For this review, take the finished solid that the model builds, in its own axes (mm). Give positions to 0.01 mm unless a question says otherwise; leave off trailing zeros.
1) For P1, Ø0.5, axis at y = 26, z = 37, coming from the -X side; P2, Ø4.5, axis at x = 104.775, z = 28.575, coming from the -Y side; P3, Ø0.5, axis at y = 26.5, z = 35.5, coming from the +X side, all flat-tipped, find the tip position at first contact; note any pin that passes through.
2) Draft analysis for pull direction X (two halves, no side actions). For faces 1 (the face through (151.107, 26.183, 28.328)), 2 (the face through (138, 25.4, 1)), state which applies: pulls with the +X half, pulls with the -X half, needs draft (parallel to the pull), parting line crosses it, or undercut.
3) Wall thickness on line 1 along Z through (x, y) = (149, 25.95); line 2 along X through (y, z) = (26.5, -28.5); line 3 along Z through (x, y) = (106.5, 26.3): over which ranges is each line inside the solid? List them lowest first.
4) We need section A-A on y = 26. Give the number of separate pieces and of enclosed holes in the cut face, and give its area (3 significant figures).
from build123d import *

# Parameters (mm, degrees)
BOSS_EXTRUDE1_DEPTH   = 25.4
SKETCH4_W             = 63.5
SKETCH4_H             = 76.2
CUT_EXTRUDE4_DEPTH    = 0.01
F_6_CLEARANCE_HOLE1_D = 3.7973
CUT_EXTRUDE5_DEPTH    = 3.5052
SKETCH8_R             = 1.89865
BOSS_EXTRUDE2_DEPTH   = 1.5875
SKETCH9_W             = 83.512513563
SKETCH9_H             = 26.66457596
CUT_EXTRUDE7_DEPTH    = 309.355274367
SKETCH10_W            = 76.2
SKETCH10_H            = 78.034990754
SKETCH10_W_2          = 120.649995745
SKETCH10_H_2          = 89.760717872
CUT_EXTRUDE8_DEPTH    = 305.02593568


with BuildPart() as part:
    # Sketch1 → Boss-Extrude1 (new body)
    with BuildSketch(Plane(origin=(0, 0, 0), x_dir=(1, 0, 0), z_dir=(0, 1, 0))):
        with BuildLine():
            Line((76.2, 38.1), (177.8, 38.1))
            add(Edge.make_bspline(
                [(177.8, -38.1), (304.8, -38.1), (304.8, 0), (304.8, 38.1), (177.8, 38.1)],
                knots=[4.71238898, 4.71238898, 4.71238898, 6.283185307, 6.283185307, 7.853981634, 7.853981634, 7.853981634], degree=2, weights=[1, 0.707106781, 1, 0.707106781, 1]))
            Line((177.8, -38.1), (76.2, -38.1))
            add(Edge.make_bspline(
                [(76.2, 38.1), (0, 38.1), (0, 0), (0, -38.1), (76.2, -38.1)],
                knots=[4.71238898, 4.71238898, 4.71238898, 6.283185307, 6.283185307, 7.853981634, 7.853981634, 7.853981634], degree=2, weights=[1, 0.707106781, 1, 0.707106781, 1]))
        make_face()
    extrude(amount=BOSS_EXTRUDE1_DEPTH)

    # Sketch4 → Cut-Extrude4 (cut)
    with BuildSketch(Plane.XZ):
        with Locations((107.95, 0)):
            Rectangle(SKETCH4_W, SKETCH4_H)
    extrude(amount=-CUT_EXTRUDE4_DEPTH, mode=Mode.SUBTRACT)

    # #6 Clearance Hole1 (through all)
    with Locations(Plane(origin=(0, 25.4, 0), x_dir=(1, 0, 0), z_dir=(0, 1, 0))):
        with Locations((104.775, 28.575), (149.225, 28.575), (149.225, -28.575), (104.775, -28.575)):
            Hole(F_6_CLEARANCE_HOLE1_D / 2)

    # Sketch7 → Cut-Extrude5 (cut)
    with BuildSketch(Plane(origin=(0, 25.4, 0), x_dir=(1, 0, 0), z_dir=(0, 1, 0))):
        Polygon((144.092356107, 28.575), (146.658678053, 24.13), (151.791321947, 24.13), (154.357643893, 28.575), (151.791321947, 33.02), (146.658678053, 33.02), align=None)
        Polygon((144.092356107, -28.575), (146.658678053, -33.02), (151.791321947, -33.02), (154.357643893, -28.575), (151.791321947, -24.13), (146.658678053, -24.13), align=None)
        Polygon((99.642356107, -28.575), (102.208678053, -33.02), (107.341321947, -33.02), (109.907643893, -28.575), (107.341321947, -24.13), (102.208678053, -24.13), align=None)
        Polygon((99.642356107, 28.575), (102.208678053, 24.13), (107.341321947, 24.13), (109.907643893, 28.575), (107.341321947, 33.02), (102.208678053, 33.02), align=None)
    extrude(amount=-CUT_EXTRUDE5_DEPTH, mode=Mode.SUBTRACT)

    # Sketch8 → Boss-Extrude2 (add)
    with BuildSketch(Plane(origin=(0, 25.4, 0), x_dir=(1, 0, 0), z_dir=(0, 1, 0))):
        with BuildLine():
            Line((76.2, 34.925), (76.2, 38.1))
            Line((76.2, 38.1), (177.8, 38.1))
            Line((177.8, 38.1), (177.8, 34.925))
            add(Edge.make_bspline(
                [(177.8, -34.925), (183.4037084, -34.925), (188.998492342, -34.813401269), (200.169898566, -34.363095557), (205.746528757, -34.024487469), (216.880255629, -33.103008305), (222.437375795, -32.520430902), (230.75625716, -31.436497802), (233.526404303, -31.040006826), (239.060480939, -30.169274267), (241.826062226, -29.694714405), (250.088902803, -28.143630441), (255.558584053, -26.942274462), (262.328557631, -25.151722447), (263.679135198, -24.778907782), (266.372677584, -24.000520191), (267.71682163, -23.594573907), (271.725857042, -22.324580042), (274.36743953, -21.409387606), (279.569151408, -19.39956311), (282.129804397, -18.306084526), (285.88296458, -16.472402408), (287.119225286, -15.828587024), (289.55372457, -14.457194234), (290.752112946, -13.729946828), (293.096789788, -12.16067691), (294.246150852, -11.316137328), (295.874693947, -9.951173652), (296.402758109, -9.47890107), (297.421867434, -8.491073847), (297.913370929, -7.974720766), (298.834097865, -6.902845016), (299.265206405, -6.34585568), (300.051083084, -5.176943461), (300.406626859, -4.564345705), (301.008906586, -3.265877479), (301.246986609, -2.597792892), (301.485043085, -1.560074348), (301.544634961, -1.206113764), (301.617830117, -0.494585391), (301.644885041, 0.214202137), (301.581423052, 0.917612733), (301.474094585, 1.618417551), (301.397802992, 1.969801613), (301.111287523, 3.001503382), (300.846416268, 3.65704054), (300.206739898, 4.920093421), (299.828668717, 5.531043925), (299.007148253, 6.686383823), (298.562585264, 7.234082094), (297.622788002, 8.284550248), (297.127404223, 8.787187569), (296.096077792, 9.756500131), (295.558527194, 10.224239157), (293.916424424, 11.566158841), (292.777517596, 12.385848353), (290.439906756, 13.923799855), (289.240807105, 14.641390764), (286.797257835, 15.999650314), (285.552669877, 16.640084306), (283.027180157, 17.859357093), (281.744712958, 18.438732265), (279.156163214, 19.543403236), (277.854905585, 20.066703794), (273.933809615, 21.564574536), (271.296832059, 22.467878334), (265.988924804, 24.133309881), (263.317871138, 24.894922167), (255.263773486, 27.00954075), (249.84032756, 28.194552175), (238.914613399, 30.236824809), (233.411910816, 31.092279963), (225.108785934, 32.171421056), (222.333695526, 32.496639974), (216.783621708, 33.081533661), (214.006661761, 33.341462159), (205.670357358, 34.029518973), (200.105614733, 34.366364864), (188.962770448, 34.814156957), (183.384662687, 34.925), (177.8, 34.925)],
                knots=[0, 0, 0, 0, 0.0625, 0.0625, 0.125, 0.125, 0.1875, 0.1875, 0.21875, 0.21875, 0.25, 0.25, 0.3125, 0.3125, 0.328125, 0.328125, 0.34375, 0.34375, 0.375, 0.375, 0.40625, 0.40625, 0.421875, 0.421875, 0.4375, 0.4375, 0.453125, 0.453125, 0.4609375, 0.4609375, 0.46875, 0.46875, 0.4765625, 0.4765625, 0.484375, 0.484375, 0.4921875, 0.4921875, 0.49609375, 0.49609375, 0.5, 0.50390625, 0.50390625, 0.5078125, 0.5078125, 0.515625, 0.515625, 0.5234375, 0.5234375, 0.53125, 0.53125, 0.5390625, 0.5390625, 0.546875, 0.546875, 0.5625, 0.5625, 0.578125, 0.578125, 0.59375, 0.59375, 0.609375, 0.609375, 0.625, 0.625, 0.65625, 0.65625, 0.6875, 0.6875, 0.75, 0.75, 0.8125, 0.8125, 0.84375, 0.84375, 0.875, 0.875, 0.9375, 0.9375, 1, 1, 1, 1], degree=3))
            Line((177.8, -34.925), (177.8, -38.1))
            Line((177.8, -38.1), (76.2, -38.1))
            Line((76.2, -38.1), (76.2, -34.925))
            add(Edge.make_bspline(
                [(76.2, 34.925), (72.560356463, 34.925), (68.943360269, 34.792561899), (61.754441862, 34.264100128), (58.182504946, 33.868162444), (51.086537454, 32.796138329), (47.562444107, 32.120418968), (40.569083399, 30.448366491), (37.099631765, 29.453110976), (32.806027277, 27.95635597), (31.949494882, 27.644206952), (30.241174952, 26.992161717), (29.390926264, 26.65279755), (26.866144113, 25.597394738), (25.212373464, 24.842354074), (21.972821409, 23.213388071), (20.386939209, 22.339638978), (17.297386897, 20.44838632), (15.793478172, 19.43129999), (13.617299122, 17.766336528), (12.904682274, 17.187440617), (11.513561893, 15.976499308), (10.840880513, 15.349552385), (9.54783147, 14.046551814), (8.927423545, 13.37053596), (8.042889277, 12.313259261), (7.755748062, 11.953602405), (7.198395375, 11.218396794), (6.928446634, 10.843070732), (5.637961842, 8.942133597), (4.781011076, 7.331767424), (4.011479694, 5.164717753), (3.872393075, 4.721427518), (3.630991775, 3.828466268), (3.528746677, 3.379752125), (3.278693467, 2.026749947), (3.187494563, 1.115610982), (3.170545544, -0.265601808), (3.185103724, -0.730659272), (3.254432294, -1.653608423), (3.308896513, -2.110722742), (3.528648511, -3.46965449), (3.750177803, -4.359086655), (4.185155464, -5.670622337), (4.348017487, -6.105682935), (4.702753212, -6.959314098), (4.89428858, -7.377540069), (5.507317523, -8.608922615), (5.967053776, -9.398893053), (6.972472791, -10.926725455), (7.518232478, -11.66454078), (8.684660756, -13.094754944), (9.299817788, -13.780178654), (11.212125162, -15.748333857), (12.581059513, -16.950990578), (14.739480167, -18.63278064), (15.476712229, -19.172714409), (16.982909755, -20.215658543), (17.753757316, -20.719762644), (20.090686263, -22.170309278), (21.683208327, -23.057695262), (26.543466505, -25.529337744), (29.892801319, -26.925597609), (35.037930237, -28.740921547), (36.773547574, -29.298627898), (39.40495658, -30.070716914), (40.286457068, -30.317183729), (42.05035166, -30.787397156), (42.933764127, -31.011448076), (47.357777286, -32.079253653), (50.919045806, -32.767054426), (58.079539287, -33.856246888), (61.678822068, -34.257202279), (68.912834907, -34.79163745), (72.5475805, -34.925), (76.2, -34.925)],
                knots=[0, 0, 0, 0, 0.0625, 0.0625, 0.125, 0.125, 0.1875, 0.1875, 0.25, 0.25, 0.265625, 0.265625, 0.28125, 0.28125, 0.3125, 0.3125, 0.34375, 0.34375, 0.375, 0.375, 0.390625, 0.390625, 0.40625, 0.40625, 0.421875, 0.421875, 0.4296875, 0.4296875, 0.4375, 0.4375, 0.46875, 0.46875, 0.4765625, 0.4765625, 0.484375, 0.484375, 0.5, 0.5, 0.5078125, 0.5078125, 0.515625, 0.515625, 0.53125, 0.53125, 0.5390625, 0.5390625, 0.546875, 0.546875, 0.5625, 0.5625, 0.578125, 0.578125, 0.59375, 0.59375, 0.625, 0.625, 0.640625, 0.640625, 0.65625, 0.65625, 0.6875, 0.6875, 0.75, 0.75, 0.78125, 0.78125, 0.796875, 0.796875, 0.8125, 0.8125, 0.875, 0.875, 0.9375, 0.9375, 1, 1, 1, 1], degree=3))
        make_face()
        with Locations(Location((149.225, 28.575, 0), (0, 0, 270))):
            Circle(SKETCH8_R, mode=Mode.SUBTRACT)
        with Locations(Location((149.225, -28.575, 0), (0, 0, 270))):
            Circle(SKETCH8_R, mode=Mode.SUBTRACT)
        with Locations(Location((104.775, -28.575, 0), (0, 0, 270))):
            Circle(SKETCH8_R, mode=Mode.SUBTRACT)
        with Locations(Location((104.775, 28.575, 0), (0, 0, 270))):
            Circle(SKETCH8_R, mode=Mode.SUBTRACT)
    extrude(amount=BOSS_EXTRUDE2_DEPTH)

    # Sketch9 → Cut-Extrude7 (cut, through all)
    with BuildSketch(Plane(origin=(0, 0, 0), x_dir=(0, 0, -1), z_dir=(1, 0, 0))):
        with Locations((0.469171425, 12.06771202)):
            Rectangle(SKETCH9_W, SKETCH9_H)
    extrude(amount=CUT_EXTRUDE7_DEPTH, mode=Mode.SUBTRACT)

    # Sketch10 → Cut-Extrude8 (cut, through all)
    with BuildSketch(Plane.XZ.offset(-25.4)):
        Rectangle(SKETCH10_W, SKETCH10_H)
        with Locations((301.624997872, -0.000109313)):
            Rectangle(SKETCH10_W_2, SKETCH10_H_2)
    extrude(amount=-CUT_EXTRUDE8_DEPTH, mode=Mode.SUBTRACT)


solid = part.part
Results list:
1. P1: stops at x = 76.2
1. P2: stops at y = 25.4
1. P3: stops at x = 177.8
2. face 1: undercut
2. face 2: needs draft
3. line 1: z = -38.1 to -30.46, -26.69 to 26.69, 30.46 to 38.1
3. line 2: x = 38.1 to 102.88, 106.67 to 147.33, 151.12 to 241.3
3. line 3: z = -38.1 to -29.37, -27.78 to 27.78, 29.37 to 38.1
4. separate pieces: 1
4. enclosed holes: 4
4. area: 14,500 mm2
